Geometry check sheet. Reference: the model listing, model coordinates, mm. A direction names the side the tool comes from. Give positions to 0.01 mm unless a question says otherwise; leave off trailing zeros. Loops run counter-clockwise (first coordinate to the right, second up) from the corner with the lowest first, then second, coordinate; pieces in that order, holes last. Notation, with made-up numbers: (73, -17.5) -> (92, -17.5) arc R33 cw to (92, 14.5) -> close; hole circle Ø5 at (-39.5, 1). An arc over 180 degrees is marked (long way). Write item = value, one per line. Start each with the question number.
```python
from build123d import *

# Parameters (mm, degrees)
F0_W      = 76.2
F0_H      = 152.4
F1_DEPTH  = 25.4
F2_T      = -2.54
F4_DEPTH  = 6.35
F6_DEPTH  = 8.89
F8_DEPTH  = 6.35
F10_DEPTH = 3.81


# Not quite as in the source:
# - a pattern or mirror of a feature is missing from the dataset's text; its kind, count and spacing are read off the source's solid


with BuildPart() as f1:
    # F0 (on Top) → F1 (new body)
    with BuildSketch(Plane.XY):
        with Locations((0, 76.2)):
            Rectangle(F0_W, F0_H)
    extrude(amount=F1_DEPTH)

    # F2
    f2_openings = [f1.faces().sort_by_distance(p)[0] for p in [
        (0, 76.2, 25.4),
    ]]
    offset(amount=F2_T, openings=f2_openings)

    # F3 (on face) → F4 (join)
    with BuildSketch(Plane.XY.offset(2.54)):
        Polygon((-6.4988862723, 57.677667588), (-22.2837403417, 45.2752783895), (-3.4451077227, 9.7248451784), (-7.3955161497, 2.54), (7.3955161497, 2.54), (3.4451077227, 9.7248451784), (22.2837403417, 45.2752783895), (6.4988862723, 57.677667588), (6.4988862723, 66.8228566647), (0, 60.9430685656), (-6.4988862723, 66.8228566647), align=None)
    extrude(amount=F4_DEPTH)

    # F5 (on face) → F6 (join)
    with BuildSketch(Plane.XY.offset(2.54)):
        Polygon((-6.4988862723, 66.8228566647), (0, 60.9430685656), (6.4988862723, 66.8228566647), (11.9773805831, 71.7794575804), (0, 85.0179677), (-11.9773805831, 71.7794575804), align=None)
    extrude(amount=F6_DEPTH)

    # F7 (on face) → F8 (join)
    with BuildSketch(Plane.XY.offset(2.54)):
        Polygon((11.9773805831, 97.4589511752), (0, 85.0179677), (11.9773805831, 71.7794575804), align=None)
        Polygon((-11.9773805831, 97.4589511752), (-11.9773805831, 71.7794575804), (0, 85.0179677), align=None)
    extrude(amount=F8_DEPTH)

    # F9 (on face) → F10 (join)
    with BuildSketch(Plane.XY.offset(2.54)):
        Polygon((-3.4451077227, 9.7248451784), (-17.0620636054, 35.4214384736), (-21.7691510916, 32.9270921648), (-8.3730621263, 10.7017857954), (-11.2379649654, 6.5747052431), (-9.2242012438, 2.7745264226), (-7.3955161497, 2.54), align=None)
    f10 = extrude(amount=F10_DEPTH)

    # F10_copies: F10 across plane
    add(f10.mirror(Plane(origin=(0, 0, 0), x_dir=(0, 0, 1), z_dir=(1, 0, 0))))


solid = f1.part
```
1) Tool access check on faces 4 (the flat face through (-1, 152.4, 13)), 5 (the flat face through (-15.165, 21.97, 4.418)). Record the directions out of +Z, -Z, +X, -X, +Y, -Y that give a thin tool (end or side, any length) a straight path to the whole face; none if there is none.
2) Thickness scan on line 1 (Y direction, x = 14, z = 14.75); line 2 (X direction, y = 45, z = 5.75); line 3 (X direction, y = 43.5, z = 9). Record the ranges inside material, lowest first.
3) Depth check by flat-ended pin: pin 1 Ø20 at (x, y) = (8, 19) entering from +Z; pin 2 Ø13 at (x, y) = (4, 82) entering from +Z; pin 3 Ø9 at (x, y) = (-16, 11.5) entering from +Z. Enter the tip coordinate at first touch or a pass-through.
4) Section check D-D (z = 14). Enter the section's corners in (x, y).
5) Section check B-B (y = 117.5). Enter the section's corners in (x, z).
6) Section check C-C (x = 20). Enter the section's corners in (y, z).
7) Draft check along X on faces 1 (the flat face through (-1, 77, 0)), 2 (the flat face through (38.1, 75, 13)), 3 (the flat face through (-14.281, 51.563, 5.671)). Enter one of: released by +X, released by -X, zero draft, split by the parting line, or undercut.
Check result:
q1.face_4 = +Z, -Z, +X, -X, +Y
q1.face_5 = +Z
q2.line_1 = 0 to 2.54, 149.86 to 152.4
q2.line_2 = -38.1 to -35.56, -22.14 to 22.14, 35.56 to 38.1
q2.line_3 = -38.1 to -35.56, 35.56 to 38.1
q3.pin_1 = 8.89
q3.pin_2 = 11.43
q3.pin_3 = 2.54
q4.outline = (-38.1, 0) -> (38.1, 0) -> (38.1, 152.4) -> (-38.1, 152.4) -> close; hole (-35.56, 2.54) -> (35.56, 2.54) -> (35.56, 149.86) -> (-35.56, 149.86) -> close
q5.outline = (-38.1, 0) -> (38.1, 0) -> (38.1, 25.4) -> (35.56, 25.4) -> (35.56, 2.54) -> (-35.56, 2.54) -> (-35.56, 25.4) -> (-38.1, 25.4) -> close
q6.outline = (0, 0) -> (152.4, 0) -> (152.4, 25.4) -> (149.86, 25.4) -> (149.86, 2.54) -> (47.07, 2.54) -> (47.07, 8.89) -> (40.97, 8.89) -> (40.97, 2.54) -> (33.86, 2.54) -> (33.86, 6.35) -> (29.99, 6.35) -> (29.99, 2.54) -> (2.54, 2.54) -> (2.54, 25.4) -> (0, 25.4) -> close
q7.face_1 = zero draft
q7.face_2 = released by +X
q7.face_3 = undercut
